Job drawing, mm, ordinate dimensions from the low corner. One solid piece. A direction names the side the tool comes from. Round coordinates to 2 decimals unless told otherwise and drop trailing zeros. Loops run counter-clockwise (first coordinate to the right, second up) from the corner with the lowest first, then second, coordinate; pieces in that order, holes last. Notation, with made-up numbers: M -34,84 L -6,84 A13 ccw -6,94 Z; hole C 35,-31.75 d5. An arc over 180 degrees is marked long. Put each result on its own line as item: value. Start each with the question number.
1) Slice it at D-D on y = 7. Give the cut face in (x, z) (3 decimals), then the cut area to 3 significant figures.
2) Drop flat-ended pins along their axis: pin 1 Ø5.5 at (x, z) = (27, 7.5) entering from -Y; pin 2 Ø3.5 at (x, z) = (25, 3) entering from +Y; pin 3 Ø15 at (x, y) = (25, 15) entering from +Z. Give the stop position or say it passes through.
3) Which spindle directions (+Z, -Z, +X, -X, +Y, -Y) get a long thin tool onto all of the face, cutting with end or side? Do the marked faces 1, 2 and 3. Say none if no direction does.
4) Slice it at C-C on x = 8. Give the cut face in (y, z).
5) Slice it at A-A on y = 12. Give the cut face in (x, z), then the cut area to 3 significant figures.
6) Slice it at B-B on z = 27. Give the cut face in (x, y), then the cut area to 3 significant figures.
7) Probe line 1 along Z through (x, y) = (26, 12); line 2 along Z through (x, y) = (12.5, 4); line 3 along Y through (x, z) = (1, 27). List the from-to ranges inside material, lowest first.
8) Pull direction Z, two halves, no side cores. Call the marked faces 4, 5 and 6: +Z half, -Z half, draft (parallel to the pull), parting line (faces both ways), or undercut.
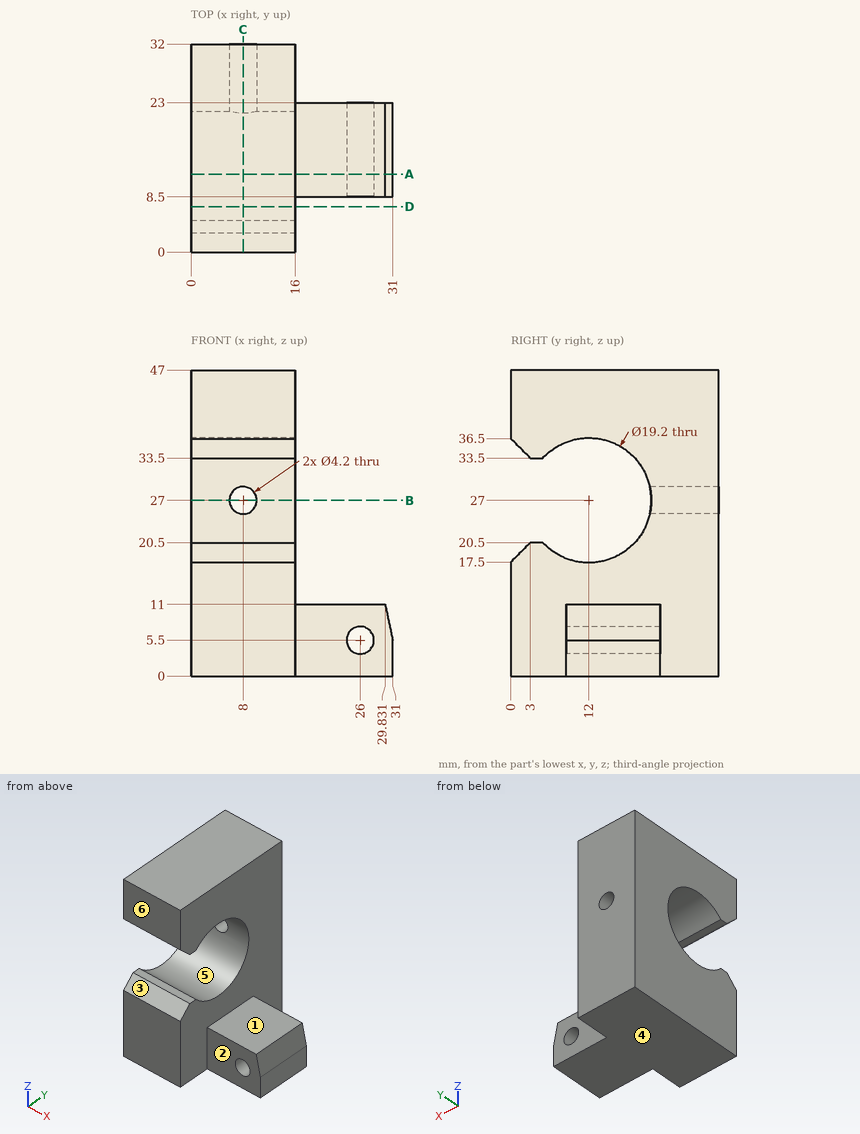
Recorded:
1. outline: M 0,0 L 16,0 L 16,18.805 L 0,18.805 Z; M 0,35.195 L 16,35.195 L 16,47 L 0,47 Z
1. area: 490 mm2
2. pin 1: stops at y = 8.5
2. pin 2: stops at y = 23
2. pin 3: stops at z = 11
3. face 1: +Z, +X, +Y, -Y
3. face 2: +Z, -Z, +X, -Y
3. face 3: +X, -X, -Y
4. outline: M 0,0 L 32,0 L 32,24.9 L 21.37,24.9 A9.6 cw 4.94,20.5 L 3,20.5 L 0,17.5 Z; M 0,36.5 L 3,33.5 L 4.94,33.5 A9.6 cw 21.37,29.1 L 32,29.1 L 32,47 L 0,47 Z
5. outline: M 0,0 L 31,0 L 31,5.5 L 29.83,11 L 16,11 L 16,17.4 L 0,17.4 Z; M 0,36.6 L 16,36.6 L 16,47 L 0,47 Z; hole C 26,5.5 d4.2
5. area: 593 mm2
6. outline: M 0,21.6 L 5.9,21.6 L 5.9,32 L 0,32 Z; M 10.1,21.6 L 16,21.6 L 16,32 L 10.1,32 Z
6. area: 123 mm2
7. line 1: z = 0 to 3.4, 7.6 to 11
7. line 2: z = 0 to 20.5, 33.5 to 47
7. line 3: y = 21.6 to 32
8. face 4: -Z half
8. face 5: undercut
8. face 6: draft
